Design review of the part shown in the three views and the two pictorial views. Dimensions are in mm from the part's minimum x, y and z. A direction names the side the tool comes from. Round coordinates to 2 decimals unless told otherwise and drop trailing zeros. Loops run counter-clockwise (first coordinate to the right, second up) from the corner with the lowest first, then second, coordinate; pieces in that order, holes last. Notation, with made-up numbers: M 5.25,26.5 L 58.25,26.5 A17 ccw 58.25,50.5 Z; hole C -32.75,35 d9. An arc over 180 degrees is marked long. Answer as CSV lines item,"result". Start each with the question number.
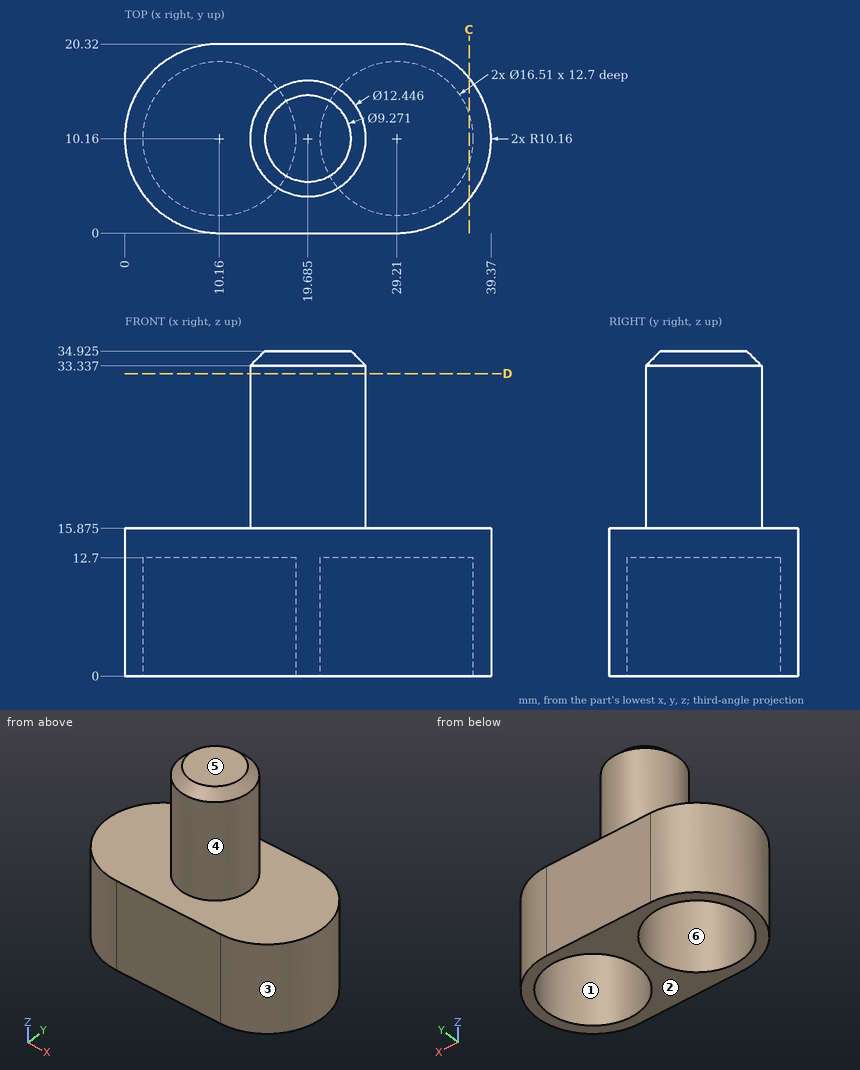
Item 1: To check wall thickness, follow line 1 (Z direction, x = 33, y = 1.5) (1 decimal); line 2 (Z direction, x = 5, y = 11.5) (1 decimal); line 3 (Y direction, x = 9, z = 9.5). State the ranges of each line that lie inside material, in increasing order.
Item 2: Tool access review of the marked faces 1 and 2: name each direction out of +Z, -Z, +X, -X, +Y, -Y from which nothing blocks a thin tool from reaching the whole face with its end or side.
Item 3: The part is to be moulded in two halves that separate along X. For the marked faces 3, 4, 5 and 6, say which applies: +X half, -X half, draft (parallel to the pull), parting line (faces both ways), or undercut.
Item 4: Consider section D-D, the plane z = 32.5. Write out the cut boundary in (x, y) (1 decimal), then the cut area to 3 significant figures.
Item 5: Insertion check: pin 1 Ø8 at (y, z) = (17, 7) entering from -X (1 decimal); pin 2 Ø4 at (y, z) = (8, 21) entering from -X; pin 3 Ø4 at (x, z) = (12.5, 31) entering from -Y. Each pin has a flat end and moves straight along its axis. Give the tip position at first contact, or say it passes through.
Item 6: Consider section C-C, the plane x = 37. Write out the cut boundary in (y, z) (1 decimal).
Found:
1,line 1,"z = 0 to 15.9"
1,line 2,"z = 12.7 to 15.9"
1,line 3,"y = 0.07 to 1.99, 18.33 to 20.25"
2,face 1,"-Z"
2,face 2,"-Z, +X, -X, +Y, -Y"
3,face 3,"+X half"
3,face 4,"parting line"
3,face 5,"draft"
3,face 6,"undercut"
4,outline,"C 19.7,10.2 d12.4"
4,area,"122 mm^2"
5,pin 1,"stops at x = 0.4"
5,pin 2,"stops at x = 13.46"
5,pin 3,"stops at y = 6.72"
6,outline,"M 3.6,0 L 7.4,0 L 7.4,12.7 L 12.9,12.7 L 12.9,0 L 16.7,0 L 16.7,15.9 L 3.6,15.9 Z"
